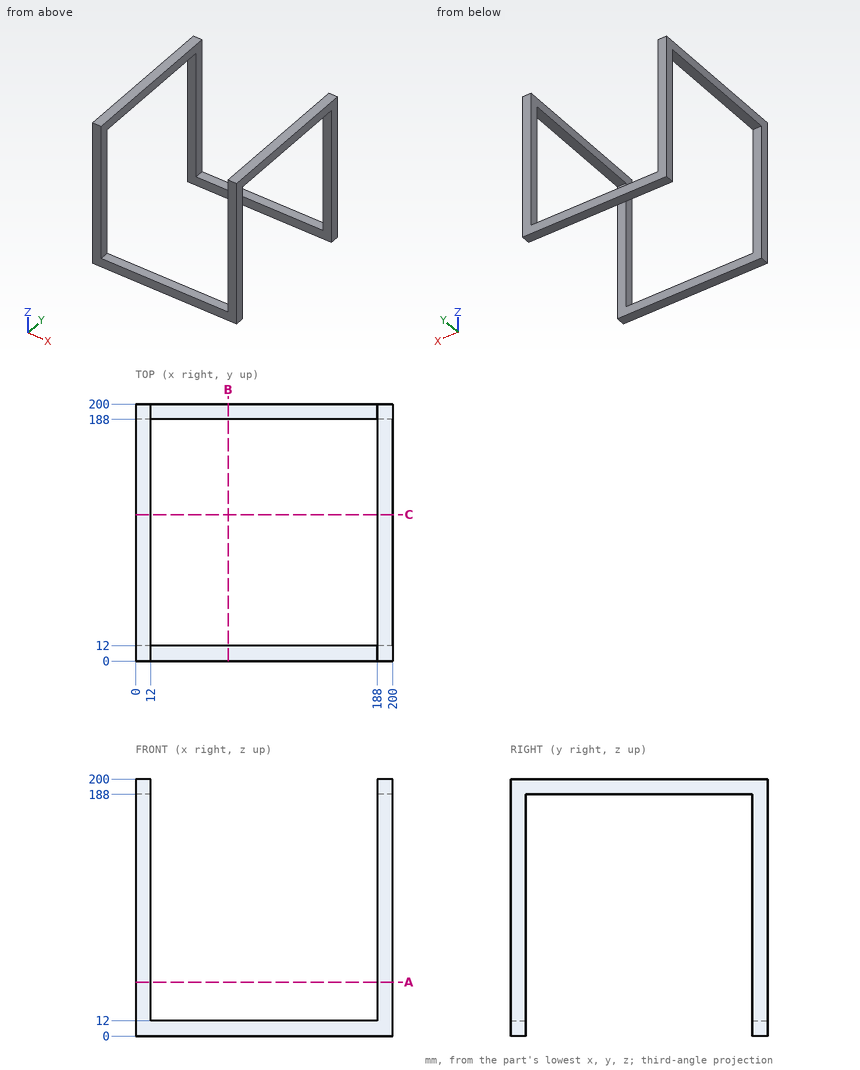
The figure shows three views and two pictorial views of one solid part (mm, origin at its lowest corner). Answer the questions. Round coordinates to 2 decimals unless told otherwise and drop trailing zeros. Order: outer loops, then holes, each group sorted by start corner. A loop starts at its lowest first (then second) coordinate and runs counter-clockwise, first axis right, second up. Notation, with made-up numbers: M 5,77.5 L 41,77.5 A13 cw 41,87.5 Z; hole C 86,-36.75 d6. An arc over 180 degrees is marked long. Put each result on its own line as item: value. Start each with the question number.
Q1. A straight line is drawn through the part: L1, parallel to Y at x = 189, z = 18. Find the intervals that lie inside material, in ascending order. Write a range as [from, to].
Q2. Section B-B, the plane x = 72 is taken. Write down the section's boundary in (y, z).
Q3. Section A-A, the plane z = 42 is taken. Write down the section's boundary in (x, y), and give its area (3 significant figures).
Q4. Section C-C, the plane y = 114 is taken. Write down the section's boundary in (x, z), and give its area (3 significant figures).
Q5. Flat-ended cylindrical pins translate along their axes: pin 1 (13 mm diameter, centred on x = 118, y = 192, fed in from +Z); pin 2 (3.5 mm diameter, centred on x = 196.5, y = 120.5, fed in from -Z). Find the tip coordinate at first contact, or state that the pin passes through.
Findings below:
1. L1: y = [0, 12], [188, 200]
2. outline: M 0,0 L 12,0 L 12,12 L 0,12 Z; M 188,0 L 200,0 L 200,12 L 188,12 Z
3. outline: M 0,0 L 12,0 L 12,12 L 0,12 Z; M 0,188 L 12,188 L 12,200 L 0,200 Z; M 188,0 L 200,0 L 200,12 L 188,12 Z; M 188,188 L 200,188 L 200,200 L 188,200 Z
3. area: 576 mm^2
4. outline: M 0,188 L 12,188 L 12,200 L 0,200 Z; M 188,188 L 200,188 L 200,200 L 188,200 Z
4. area: 288 mm^2
5. pin 1: stops at z = 12
5. pin 2: stops at z = 188
